Verification items for the finished model (mm, model axes). Face numbers are marked on the shaded views. A direction names the side the tool comes from. Coordinates: 2 decimals unless noted, no trailing zeros. Write each loop counter-clockwise with the first axis right and the second up, starting at its lowest first coordinate (ties: lowest second). Pieces come first, ordered by that corner, then holes. Notation, with made-up numbers: (39.25, -32) -> (76.25, -32) arc R22 ccw to (76.25, -24) -> close; hole circle Ø8 at (-26, 74.25). An arc over 180 degrees is marked (long way). Answer in a Markdown table with one row per item.
```python
from build123d import *

# Parameters (mm, degrees)
F1_DEPTH = 30
F3_DEPTH = 12.5
F4_R     = 2
F5_R     = 2
F6_DEPTH = 10
F7_R     = 2.5
F7_R_2   = 2
F8_DEPTH = 2


with BuildPart() as f1:
    # F0 (on Front) → F1 (new body)
    with BuildSketch(Plane.XZ):
        with BuildLine():
            ThreePointArc((-8, 203.042459), (0, 203.2), (8, 203.042459))
            Line((8, 203.042459), (5, 216.2))
            Line((5, 216.2), (0, 218.2))
            Line((0, 218.2), (-5, 216.2))
            Line((-5, 216.2), (-8, 203.042459))
        make_face()
    extrude(amount=-F1_DEPTH)

    # F2 (on Right) → F3 (cut, symmetric)
    with BuildSketch(Plane.YZ):
        Polygon((30, 203.042459), (30, 218.2), (27, 218.2), align=None)
    extrude(amount=F3_DEPTH, both=True, mode=Mode.SUBTRACT)

    # F4
    f4_edges = [f1.edges().sort_by_distance(p)[0] for p in [
        (5, 13.697921, 216.2),
        (0, 13.5, 218.2),
        (-5, 13.697921, 216.2),
        (-6.5, 28.697921, 209.621229),
        (-2.5, 27.197921, 217.2),
        (6.5, 28.697921, 209.621229),
    ]]
    fillet(f4_edges, radius=F4_R)

    # F5 (on face) → F6 (cut)
    with BuildSketch(Plane.XZ):
        with Locations((0, 214.045934)):
            Circle(F5_R)
    extrude(amount=-F6_DEPTH, mode=Mode.SUBTRACT)

    # F7 (on face) → F8 (join)
    with BuildSketch(Plane.XZ):
        with Locations((0, 214.045934)):
            Circle(F7_R)
        with Locations((0, 214.045934)):
            Circle(F7_R_2, mode=Mode.SUBTRACT)
    extrude(amount=F8_DEPTH)


solid = f1.part
```
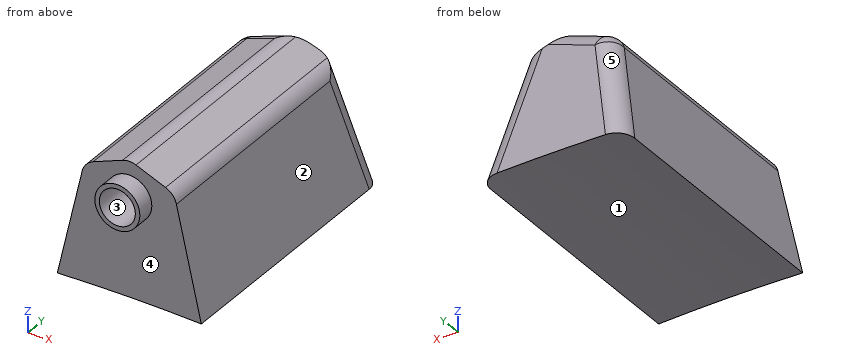
1. Access from +Z, -Z, +X, -X, +Y, -Y to the whole of each face (thin tool, end or side, straight path). Record for the marked faces 1 and 2.
Findings below:
| item | result |
|---|---|
| face 1 | -Z, +Y, -Y |
| face 2 | +Z, +X, +Y, -Y |
2. Sectioned sample at B-B, the plane y = 2. Record the cut outline in (x, z), and give its area (3 significant figures).
Findings below:
| item | result |
|---|---|
| outline | (-8, 203.04) arc R203.2 cw to (8, 203.04) -> (5.23, 215.18) arc R2 ccw to (4.03, 216.59) -> (0.74, 217.9) arc R2 ccw to (-0.74, 217.9) -> (-4.03, 216.59) arc R2 ccw to (-5.23, 215.18) -> close; hole circle Ø4 at (0, 214.05) |
| area | 166 mm² |
3. Sectioned sample at A-A, the plane y = 23. Record the cut outline in (x, z), and give its area (3 significant figures).
Findings below:
| item | result |
|---|---|
| outline | (-8, 203.04) arc R203.2 cw to (8, 203.04) -> (5.23, 215.18) arc R2 ccw to (4.03, 216.59) -> (0.74, 217.9) arc R2 ccw to (-0.74, 217.9) -> (-4.03, 216.59) arc R2 ccw to (-5.23, 215.18) -> close |
| area | 179 mm² |
4. Material ranges on probe 1 along Z at (x, y) = (0, 5); probe 2 along Y at (x, z) = (-1.5, 216.5); probe 3 along Y at (x, z) = (-5, 212), recorded low to high. Write a range as from..to.
Findings below:
| item | result |
|---|---|
| probe 1 | z = 203.2..212.05, 216.05..218.05 |
| probe 2 | y = 0..27.23 |
| probe 3 | y = 0..27.96 |
5. Go/stop test with flat-tipped pins: pin 1 (5 mm diameter, centred on y = 14.5, z = 212, fed in from -X); pin 2 (5 mm diameter, centred on y = 21, z = 216.5, fed in from -X); pin 3 (8 mm diameter, centred on y = 17, z = 206, fed in from -X). Record where each tip stops, or that it passes through.
Findings below:
| item | result |
|---|---|
| pin 1 | stops at x = -6.53 |
| pin 2 | stops at x = -5.5 |
| pin 3 | stops at x = -8 |
6. Release check for a two-part mould opening along X. For the marked faces 3, 4 and 5 record: released by +X, released by -X, zero draft, split by the parting line, or undercut.
Findings below:
| item | result |
|---|---|
| face 3 | undercut |
| face 4 | zero draft |
| face 5 | released by -X |
